from build123d import *

# Parameters (mm, degrees)
SKETCH_R     = 26
PAD_DEPTH    = 20
SKETCH001_R  = 3.25
POCKET_DEPTH = 55
CHAMFER_SIZE = 1.5


with BuildPart() as part:
    # Sketch → Pad (new body, symmetric)
    with BuildSketch(Plane.XY):
        Polygon((-45, 0), (45, 0), (45, 10), (43, 10), (43, 54), (27.5, 54), (13.5, 68), (-13.5, 68), (-27.5, 54), (-43, 54), (-43, 10), (-45, 10), align=None)
        with Locations((0, 34)):
            Circle(SKETCH_R, mode=Mode.SUBTRACT)
    extrude(amount=PAD_DEPTH, both=True)

    # Sketch001 (on Face1 of Pad) → Pocket (cut)
    with BuildSketch(Plane.XZ):
        with Locations((-35, 10)):
            Circle(SKETCH001_R)
        with Locations((35, 10)):
            Circle(SKETCH001_R)
        with Locations((35, -10)):
            Circle(SKETCH001_R)
        with Locations((-35, -10)):
            Circle(SKETCH001_R)
    extrude(amount=-POCKET_DEPTH, mode=Mode.SUBTRACT)

    # Chamfer
    chamfer_edges = [part.edges().sort_by_distance(p)[0] for p in [
        (45, 10, 0),
        (-45, 10, 0),
        (-43, 54, 0),
        (43, 54, 0),
    ]]
    chamfer(chamfer_edges, length=CHAMFER_SIZE)


solid = part.part
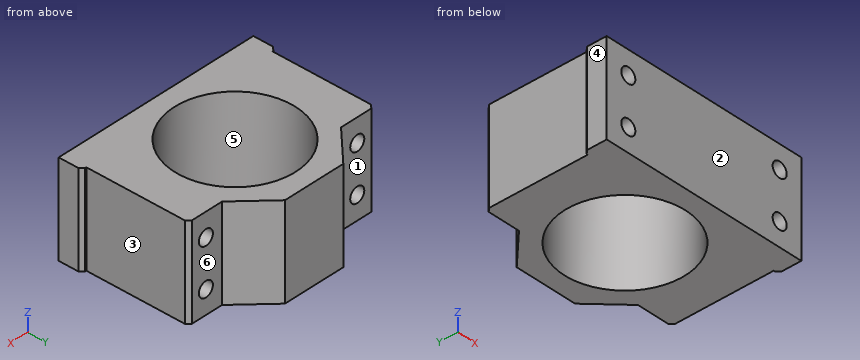
CAD build for the part. Positions are in the model's coordinates, mm. Face numbers are marked on the shaded views. A direction names the side the tool comes from. Coordinates: 2 decimals unless noted, no trailing zeros. Loops run counter-clockwise (first coordinate to the right, second up) from the corner with the lowest first, then second, coordinate; pieces in that order, holes last. Notation, with made-up numbers: (64, 10) - (76, 10) arc R26 cw to (76, 40) - close; hole circle Ø9 at (89, 38). An arc over 180 degrees is marked (long way). Use one line per item in the form item = value. Start each with the question number.
1) Flat gauge pins, fed straight in: pin 1 (4 mm diameter, centred on x = 37, z = 8, fed in from +Y); pin 2 (5 mm diameter, centred on y = 53.5, z = -15, fed in from -X); pin 3 (11 mm diameter, centred on x = -31, z = -6, fed in from +Y); pin 4 (4 mm diameter, centred on x = 7.5, z = -1, fed in from -Y). Where does each tip first touch, or does it go through?
2) Band-saw the part on B-B (y = 34). Give the cut face in (x, z).
3) Two-plate mould, pull along X, no slides. Class the marked faces 4, 5 and 6: +X half, -X half, draft (parallel to the pull), parting line (faces both ways), or undercut.
4) Band-saw the part on C-C (x = 0). Give the cut face in (y, z).
5) Drill centre lines: L1, parallel to Z at x = 35, y = 12; L2, parallel to X at y = 4, z = -7; L3, parallel to Z at x = -32, y = 26.5. Where is each one in solid material? Low to high. Write a range as from..to.
6) Band-saw the part on A-A (z = -10). Give the cut face in (x, y), and give its area (3 significant figures).
7) Band-saw the part on D-D (z = 2). Give the cut face in (x, y), and give its area (3 significant figures).
8) Tool access for the marked faces 1, 2 and 3: list every direction of +Z, -Z, +X, -X, +Y, -Y with a clear straight run to the whole face (end or side of a thin tool).
Check values:
q1.pin_1 = 54
q1.pin_2 = -43
q1.pin_3 = 56
q1.pin_4 = 0
q2.outline = (-43, -20) - (-26, -20) - (-26, 20) - (-43, 20) - close; (26, -20) - (43, -20) - (43, 20) - (26, 20) - close; hole circle Ø6.5 at (-35, -10); hole circle Ø6.5 at (-35, 10); hole circle Ø6.5 at (35, -10); hole circle Ø6.5 at (35, 10)
q3.face_4 = -X half
q3.face_5 = undercut
q3.face_6 = draft
q4.outline = (0, -20) - (8, -20) - (8, 20) - (0, 20) - close; (60, -20) - (68, -20) - (68, 20) - (60, 20) - close
q5.L1 = -20..-13.25, -6.75..6.75, 13.25..20
q5.L2 = -45..-36.25, -33.75..33.75, 36.25..45
q5.L3 = -20..-11.25, -8.75..8.75, 11.25..20
q6.outline = (-45, 0) - (-38.25, 0) - (-38.25, 54) - (-41.5, 54) - (-43, 52.5) - (-43, 10) - (-43.5, 10) - (-45, 8.5) - close; (-31.75, 0) - (31.75, 0) - (31.75, 54) - (27.5, 54) - (13.5, 68) - (-13.5, 68) - (-27.5, 54) - (-31.75, 54) - close; (38.25, 0) - (45, 0) - (45, 8.5) - (43.5, 10) - (43, 10) - (43, 52.5) - (41.5, 54) - (38.25, 54) - close; hole circle Ø52 at (0, 34)
q6.area = 2,430 mm2
q7.outline = (-45, 0) - (45, 0) - (45, 8.5) - (43.5, 10) - (43, 10) - (43, 52.5) - (41.5, 54) - (27.5, 54) - (13.5, 68) - (-13.5, 68) - (-27.5, 54) - (-41.5, 54) - (-43, 52.5) - (-43, 10) - (-43.5, 10) - (-45, 8.5) - close; hole circle Ø52 at (0, 34)
q7.area = 3,130 mm2
q8.face_1 = +Z, -Z, -X, +Y
q8.face_2 = +Z, -Z, +X, -X, -Y
q8.face_3 = +Z, -Z, +X, +Y
